For this review, take the finished solid that the model builds, in its own axes (mm). A direction names the side the tool comes from. Coordinates: 2 decimals unless noted, no trailing zeros. Loops run counter-clockwise (first coordinate to the right, second up) from the corner with the lowest first, then second, coordinate; pieces in that order, holes last. Notation, with made-up numbers: M 44,8.5 L 59,8.5 A12 cw 59,27.5 Z; hole C -6,66.25 d7. An arc over 180 degrees is marked long. Put each result on its own line as item: value.
```python
from build123d import *

# Parameters (mm, degrees)
F1_R      = 3
F2_DEPTH  = 7.5
F3_R      = 3
F4_DEPTH  = 3
F5_R      = 2
F6_DEPTH  = 2
F7_SIZE2  = 1.99999
F7_SIZE   = 1.49999
F8_D      = 0.4
F10_D     = 2.5
F10_DEPTH = 5
F10_TIP   = 0.7510757738


# Not quite as in the source:
# - a fillet or chamfer is up to 0.001 mm smaller than in the source, because OpenCascade refuses the exact size


with BuildPart() as f2:
    # F1 (on face) → F2 (new body)
    with BuildSketch(Plane.XY):
        Circle(F1_R)
    extrude(amount=F2_DEPTH)

    # F3 (on face) → F4 (join)
    with BuildSketch(Plane.XY.offset(7.5)):
        Polygon((3.5, -2.0207259422), (3.5, 2.0207259422), (0, 4.0414518843), (-3.5, 2.0207259422), (-3.5, -2.0207259422), (0, -4.0414518843), align=None)
        Circle(F3_R, mode=Mode.SUBTRACT)
        Circle(F3_R)
    extrude(amount=F4_DEPTH)

    # F5 (on face) → F6 (join)
    with BuildSketch(Plane.XY.offset(10.5)):
        Circle(F5_R)
    extrude(amount=F6_DEPTH)

    # F7 (size 1.5 and 2 in the source; OpenCascade refuses exactly that, so slightly less here)
    f7_edges = [f2.edges().sort_by_distance(p)[0] for p in [
        (-2, 0, 12.5),
    ]]
    f7_side = f2.faces().sort_by_distance((0, 0, 12.5))[0]
    chamfer(f7_edges, length=F7_SIZE, length2=F7_SIZE2, reference=f7_side)

    # F8 (through all)
    with Locations(Plane(origin=(0, 0, 0), x_dir=(1, 0, 0), z_dir=(0, 0, -1))):
        with Locations((0, 0)):
            Hole(F8_D / 2)

    # F10
    with Locations(Plane(origin=(0, 0, 0), x_dir=(1, 0, 0), z_dir=(0, 0, -1))):
        with Locations((0, 0)):
            Hole(F10_D / 2, depth=F10_DEPTH)
            with Locations((0, 0, -(F10_DEPTH + F10_TIP / 2))):  # 118° drill point
                Cone(0, F10_D / 2, F10_TIP, mode=Mode.SUBTRACT)


solid = f2.part
```
(1) Draft analysis for pull direction Y (two halves, no side actions). For faces 1 (the cylindrical face through (0.27, 1.22, 2.54)), 2 (the flat face through (1.8, 3, 9)), 3 (the flat face through (3.5, 0, 9)), state which applies: +Y half, -Y half, draft (parallel to the pull), parting line (faces both ways), or undercut.
Determined:
face 1: undercut
face 2: +Y half
face 3: draft
(2) Wall thickness on line 1 along Y through (x, z) = (0, 3.5); line 2 along Z through (x, y) = (1.5, -1.5); line 3 along X through (y, z) = (-0.5, 1.5): over which ranges is each line inside the solid? List them lowest first. Write a range as [from, to].
Determined:
line 1: y = [-3, -1.25], [1.25, 3]
line 2: z = [0, 10.5]
line 3: x = [-2.96, -1.15], [1.15, 2.96]
(3) For pin 1 (1.5 mm diameter, centred on x = -2.5, z = 3.5, fed in from -Y); pin 2 (4 mm diameter, centred on x = -1, z = 2, fed in from -Y); pin 3 (4 mm diameter, centred on x = -2.5, y = -2.5, fed in from +Z), all flat-tipped, find the tip position at first contact; note any pin that passes through.
Determined:
pin 1: stops at y = -2.44
pin 2: stops at y = -3
pin 3: stops at z = 11.12
(4) Add section B-B (z = 8.5). Write out the cut boundary in (x, y), plus the area to 3 significant figures.
Determined:
outline: M -3.5,-2.02 L 0,-4.04 L 3.5,-2.02 L 3.5,2.02 L 0,4.04 L -3.5,2.02 Z; hole C 0,0 d0.4
area: 42.3 mm^2
(5) Add section D-D (x = 2.5). Write out the cut boundary in (y, z).
Determined:
outline: M -2.6,7.5 L -1.66,7.5 L -1.66,0 L 1.66,0 L 1.66,7.5 L 2.6,7.5 L 2.6,10.5 L -2.6,10.5 Z
(6) Add section C-C (y = 2.25). Write out the cut boundary in (x, z), plus the area to 3 significant figures.
Determined:
outline: M -3.1,7.5 L -1.98,7.5 L -1.98,0 L 1.98,0 L 1.98,7.5 L 3.1,7.5 L 3.1,10.5 L -3.1,10.5 Z
area: 48.4 mm^2
(7) Tool access review of faces 4 (the flat face through (-2, -2, 10.5)), 5 (the flat face through (-1.726, 3.045, 8.979)), 6 (the cylindrical face through (-3, 0, 4)): name each direction out of +Z, -Z, +X, -X, +Y, -Y from which nothing blocks a thin tool from reaching the whole face with its end or side.
Determined:
face 4: +Z
face 5: +Z, -Z, -X, +Y
face 6: -Z
